Here's how the part is built. I have some questions about the finished solid (model axes, mm). A direction names the side the tool comes from. Coordinates: 2 decimals unless noted, no trailing zeros. Write each loop counter-clockwise with the first axis right and the second up, starting at its lowest first coordinate (ties: lowest second). Pieces come first, ordered by that corner, then holes.
Item 1: We'd pull the mould along Z, two halves only. Please class faces 4 (the face through (-20.13, -15.44, 144.38)), 5 (the face through (-3.645, 27.763, 144.05)), 6 (the face through (0, 0, 0)): +Z half, -Z half, draft (parallel to the pull), parting line (faces both ways), or undercut.
Item 2: If I drill on line 1 (Y direction, x = 0, z = 76); line 2 (Z direction, x = -4, y = -14); line 3 (Z direction, x = 6, y = -2), over which ranges is the centre line in solid material (lowest first)?
Item 3: For faces 1 (the face through (-6.065, -27.314, 144.463)), 2 (the face through (-5.558, -25.029, 0.302)), 3 (the face through (1.31, -0.78, 144.399)), which set-ups out of +Z, -Z, +X, -X, +Y, -Y let a thin tool reach every point of the face, with its end or its side?
Item 4: I'm going to push flat-ended pins straight in: pin 1 Ø2 at (x, y) = (-8, 20) entering from +Z; pin 2 Ø1.5 at (x, z) = (19.5, 69) entering from -Y; pin 3 Ø0.5 at (x, z) = (6, 144) entering from +Y; pin 4 Ø1 at (x, y) = (-12, -10.5) entering from -Z. Where does each tip first touch, or does it pass through?
Item 5: If we section it at A-A (z = 92.5): Please give me the cut outline in (x, y).
from build123d import *

# Parameters (mm, degrees)
F2_R      = 29.21
F4_R      = 29.21
F0_R      = 25.4
F8_R      = 27.94
F11_R     = 28.575
F13_T     = -2.54
F15_R     = 27.94
F16_DEPTH = 0.762
F18_DEPTH = 0.635


with BuildPart() as f5:
    # F2 (on offset) → F5 section 0
    with BuildSketch(Plane.XY.offset(4.826)):
        Circle(F2_R)
    # F4 (on offset) → F5 section 1
    with BuildSketch(Plane.XY.offset(139.7)):
        Circle(F4_R)
    loft()

    # F0 (on Top) → F6 section 0
    with BuildSketch(Plane.XY):
        Circle(F0_R)
    # F2 (on offset) → F6 section 1
    with BuildSketch(Plane.XY.offset(4.826)):
        Circle(F2_R)
    loft()

    # F4 (on offset) → F9 section 0
    with BuildSketch(Plane.XY.offset(139.7)):
        Circle(F4_R)
    # F8 (on offset) → F9 section 1
    with BuildSketch(Plane.XY.offset(144.272)):
        Circle(F8_R)
    loft()

    # F8 (on offset) → F12 section 0
    with BuildSketch(Plane.XY.offset(144.272)):
        Circle(F8_R)
    # F11 (on offset) → F12 section 1
    with BuildSketch(Plane.XY.offset(147.32)):
        Circle(F11_R)
    loft()

    # F13
    f13_openings = [f5.faces().sort_by_distance(p)[0] for p in [
        (0, 0, 147.32),
    ]]
    offset(amount=F13_T, openings=f13_openings, kind=Kind.INTERSECTION)

    # F15 (on offset) → F16 (join)
    with BuildSketch(Plane.XY.offset(143.764)):
        Circle(F15_R)
        with BuildLine():
            add(Edge.make_bspline(
                [(8.9813927189, -5.08), (10.307283956, -7.660759653), (15.5638091176, -11.3190362963), (24.5819782778, 0.156554303), (16.2046906326, 9.5661078257), (10.4008527308, 7.3320350733), (8.9813927189, 5.08)],
                knots=[0, 0, 0, 0, 0.1793099128, 0.3991725973, 0.6069429862, 0.7863905321, 0.7863905321, 0.7863905321, 0.7863905321], degree=3))
            add(Edge.make_bspline(
                [(8.9813927189, 5.08), (7.2917062072, 2.3992388266), (7.4018764658, -2.0055760179), (8.9813927189, -5.08)],
                knots=[0.7863905321, 0.7863905321, 0.7863905321, 0.7863905321, 1, 1, 1, 1], degree=3))
        make_face(mode=Mode.SUBTRACT)
        with BuildLine():
            add(Edge.make_bspline(
                [(8.9813927189, 5.08), (7.2917062072, 2.3992388266), (7.4018764658, -2.0055760179), (8.9813927189, -5.08)],
                knots=[0.7863905321, 0.7863905321, 0.7863905321, 0.7863905321, 1, 1, 1, 1], degree=3))
            Line((8.9813927189, -5.08), (8.9813927189, 0))
            Line((8.9813927189, 0), (8.9813927189, 5.08))
        make_face()
    extrude(amount=-F16_DEPTH)

    # F17 (on offset) → F18 (join)
    with BuildSketch(Plane.XY.offset(143.764)):
        with BuildLine():
            Line((11.6892714785, -6.35), (11.6892714785, 0))
            Line((11.6892714785, 0), (11.6892714785, 6.35))
            Line((11.6892714785, 6.35), (0, 6.35))
            add(Edge.make_bspline(
                [(0, -6.35), (1.8282559625, -4.4581892492), (1.6638111749, 4.50159086), (0, 6.35)],
                knots=[0.8311304713, 0.8311304713, 0.8311304713, 0.8311304713, 1, 1, 1, 1], degree=3))
            Line((0, -6.35), (11.6892714785, -6.35))
        make_face()
        with BuildLine():
            add(Edge.make_bspline(
                [(0, -6.35), (1.8282559625, -4.4581892492), (1.6638111749, 4.50159086), (0, 6.35)],
                knots=[0.8311304713, 0.8311304713, 0.8311304713, 0.8311304713, 1, 1, 1, 1], degree=3))
            add(Edge.make_bspline(
                [(0, 6.35), (-0.8350152674, 7.2776592654), (-3.4873611567, 5.389008621), (-7.2168226702, 8.4501082119), (-13.9400747086, 7.2984183342), (-13.0107401815, -0.2357314092), (-14.5251656567, -4.4878007238), (-8.0963607859, -10.2798866877), (-4.5226600604, -4.9183886243), (-1.0424695397, -7.4287084101), (0, -6.35)],
                knots=[0, 0, 0, 0, 0.0847503832, 0.1853664744, 0.2931999501, 0.4132443298, 0.5139191398, 0.6328846388, 0.7348412518, 0.8311304713, 0.8311304713, 0.8311304713, 0.8311304713], degree=3))
        make_face()
        with BuildLine():
            add(Edge.make_bspline(
                [(0, 4.6740733087), (-1.0550088408, 5.935167024), (-4.791474758, 5.2358502182), (-7.4773661307, 0.0019184091), (-4.9055168376, -5.0690387184), (1.6043119196, -6.306676079), (1.5736327616, 2.7930479473), (0, 4.6740733087)],
                knots=[0, 0, 0, 0, 0.1740799793, 0.3708117314, 0.5638311353, 0.7403453431, 1, 1, 1, 1], degree=3))
        make_face(mode=Mode.SUBTRACT)
    extrude(amount=F18_DEPTH)


solid = f5.part
Answer list:
1. face 4: +Z half
1. face 5: undercut
1. face 6: -Z half
2. line 1: y = -29.21 to -26.67, 26.67 to 29.21
2. line 2: z = 0 to 2.54, 143 to 143.76
2. line 3: z = 0 to 2.54, 143 to 144.4
3. face 1: none
3. face 2: -Z
3. face 3: +Z
4. pin 1: stops at z = 143.76
4. pin 2: stops at y = -22.4
4. pin 3: stops at y = 27.45
4. pin 4: stops at z = 0
5. outline: circle Ø58.42 at (0, 0); hole circle Ø53.34 at (0, 0)
